Design review of the part built by this model. Coordinates are the model's own, in mm. Face numbers are marked on the shaded views. Round coordinates to 2 decimals unless told otherwise and drop trailing zeros. Loops run counter-clockwise (first coordinate to the right, second up) from the corner with the lowest first, then second, coordinate; pieces in that order, holes last. Notation, with made-up numbers: (80.25, -33) - (99.25, -33) arc R16 cw to (99.25, -21) - close; hole circle Ø8 at (60, 23.5). An arc over 180 degrees is marked (long way). Return JSON: item names as keys, results as strings. Group by question number.
(1) We need section A-A, the plane y = 15. Write out the cut boundary in (x, z), and give its area (3 significant figures).
(2) We need section C-C, the plane z = 45. Write out the cut boundary in (x, y), and give its area (3 significant figures).
(3) We need section D-D, the plane z = -32. Write out the cut boundary in (x, y), and give its area (3 significant figures).
(4) Wall thickness on L1, parallel to Z at x = 0.6, y = 30; L2, parallel to Y at x = 0.5, z = 45; L3, parallel to Z at x = 1.5, y = 17.5: over which ranges is each line inside the solid? List them lowest first. Write a range as [from, to].
(5) We need section B-B, the plane z = 20. Write out the cut boundary in (x, y), and give its area (3 significant figures).
(6) Clearance check with flat-ended pins moving along their axes: pin 1 (4 mm diameter, centred on x = 5, y = 60, fed in from +Z); pin 2 (16.5 mm diameter, centred on y = 18.5, z = -22, fed in from +X); pin 3 (4 mm diameter, centred on x = 1.5, z = 45.5, fed in from +Y); pin 4 (5 mm diameter, centred on x = 6, z = 28.5, fed in from +Y). State where each tip first meets the part, or that it passes through.
(7) The part is to be moulded in two halves that separate along X. For the marked faces 1, 2 and 3, say which applies: pulls with the +X half, pulls with the -X half, needs draft (parallel to the pull), parting line crosses it, or undercut.
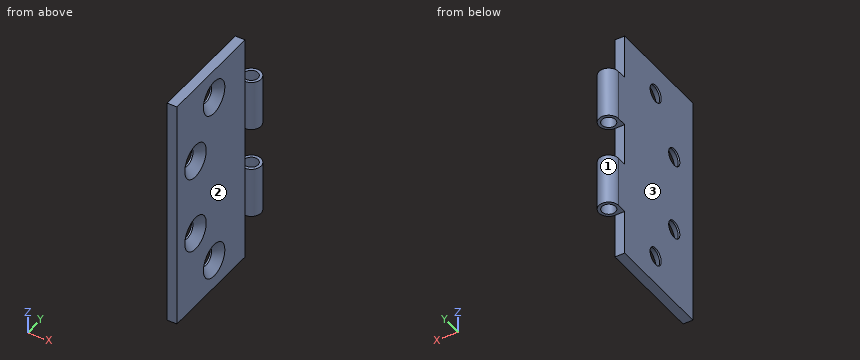
from build123d import *

# Parameters (mm, degrees)
SKETCH_1_W                 = 5
SKETCH_1_H                 = 60
EXTRUDE_1_DEPTH            = 60
SKETCH_2_R                 = 5
SKETCH_4_R                 = 3.5
CUT_EXTRUDE_1_DEPTH        = 137.839321834
HOLE_WIZARD_M81_AT_2_COUNT = 2
HOLE_WIZARD_M81_AT_2_PITCH = 29.154759474
CUT_EXTRUDE_2_DEPTH        = 89.600225733
CUT_EXTRUDE_2_DEPTH_BACK   = 89.600225733
SKETCH_7_W                 = 23
SKETCH_7_H                 = 10
SKETCH_7_W_2               = 22


with BuildPart() as part:
    # Эскиз1 → Вытянуть-Тонкостенный1 (new, symmetric)
    with BuildSketch(Plane.XY):
        with Locations((2.5, 30)):
            Rectangle(SKETCH_1_W, SKETCH_1_H)
    extrude(amount=EXTRUDE_1_DEPTH, both=True)

    # По траектории1: sweep along a curve in space
    with BuildLine() as sweep_1_path:
        Line((5, 60, 60), (5, 60, -60))
    # Эскиз2 → По траектории1 (sweep)
    with BuildSketch(Plane.XY.offset(60)):
        with Locations((5, 60)):
            Circle(SKETCH_2_R)
    sweep(path=sweep_1_path.line)

    # Эскиз4 → Вырез-Вытянуть1 (cut, through all)
    with BuildSketch(Plane.XY.offset(60)):
        with Locations((5, 60)):
            Circle(SKETCH_4_R)
    extrude(amount=-CUT_EXTRUDE_1_DEPTH, mode=Mode.SUBTRACT)

    # Эскиз5 → Зенковка для  винта с плоской головкой M81 (revolve, cut)
    with BuildSketch(Plane(origin=(5, 30, 45), x_dir=(0, 0, -1), z_dir=(0, 1, 0))):
        Polygon((0, 0), (0, 5), (4.5, 5), (4.5, 4.15), (8.65, 0), align=None)
    hole_wizard_m81 = revolve(axis=Axis((11.35, 30, 45), (-1, 0, 0)), mode=Mode.SUBTRACT)

    # Зенковка для  винта с плоской головкой M81 at 2: Зенковка для  винта с плоской головкой M81 ×2
    with Locations(*[Vector(0, -0.5144957554275265, -0.8574929257125442) * (i * HOLE_WIZARD_M81_AT_2_PITCH) for i in range(1, HOLE_WIZARD_M81_AT_2_COUNT)]):
        add(hole_wizard_m81, mode=Mode.SUBTRACT)

    # Зеркальное отражение1: Зенковка для  винта с плоской головкой M81 across plane
    add(hole_wizard_m81.mirror(Plane.XY), mode=Mode.SUBTRACT)

    # Зеркальное отражение1 copy 1 sketch → Зеркальное отражение1 copy 1 (revolve, cut)
    with BuildSketch(Plane(origin=(5, 15, -20), x_dir=(0, 0, 1), z_dir=(0, 1, 0))):
        Polygon((0, 0), (0, -5), (4.5, -5), (4.5, -4.15), (8.65, 0), align=None)
    revolve(axis=Axis((11.35, 15, -20), (1, 0, 0)), mode=Mode.SUBTRACT)

    # Эскиз7 → Вырез-Вытянуть2 (cut, two sides: drawn at the far end of the back side and taken through both)
    with BuildSketch(Plane(origin=(5, 0, 0), x_dir=(0, 0, -1), z_dir=(1, 0, 0)).offset(-CUT_EXTRUDE_2_DEPTH_BACK)):
        with Locations((48.5, 60)):
            Rectangle(SKETCH_7_W, SKETCH_7_H)
        with Locations((0, 60)):
            Rectangle(SKETCH_7_W_2, SKETCH_7_H)
        with Locations((-48.5, 60)):
            Rectangle(SKETCH_7_W, SKETCH_7_H)
    extrude(amount=CUT_EXTRUDE_2_DEPTH + CUT_EXTRUDE_2_DEPTH_BACK, mode=Mode.SUBTRACT)


solid = part.part
Solutions:
{
 "1": {"outline": "(0, -60) - (5, -60) - (5, -28.65) - (0.85, -24.5) - (0, -24.5) - close; (0, -15.5) - (0.85, -15.5) - (5, -11.35) - (5, 11.35) - (0.85, 15.5) - (0, 15.5) - close; (0, 24.5) - (0.85, 24.5) - (5, 28.65) - (5, 60) - (0, 60) - close", "area": "476 mm^2"},
 "2": {"outline": "(0, 0) - (5, 0) - (5, 21.35) - (0.85, 25.5) - (0, 25.5) - close; (0, 34.5) - (0.85, 34.5) - (5, 38.65) - (5, 55) - (0, 55) - close", "area": "213 mm^2"},
 "3": {"outline": "(0, 0) - (5, 0) - (5, 55) arc R5 ccw (long way) to (0, 60) - close; hole circle Ø7 at (5, 60)", "area": "320 mm^2"},
 "4": {"L1": "[-60, -49.5], [-40.5, 40.5], [49.5, 60]", "L2": "[0, 25.5], [34.5, 55]", "L3": "[-60, -24.5], [-15.5, 15.5], [24.5, 60]"},
 "5": {"outline": "(0, 0) - (5, 0) - (5, 6.35) - (0.85, 10.5) - (0, 10.5) - close; (0, 19.5) - (0.85, 19.5) - (5, 23.65) - (5, 55) arc R5 ccw (long way) to (0, 60) - close; hole circle Ø7 at (5, 60)", "area": "258 mm^2"},
 "6": {"pin 1": "through", "pin 2": "x = 5", "pin 3": "y = 55", "pin 4": "y = 65"},
 "7": {"face 1": "parting line crosses it", "face 2": "pulls with the +X half", "face 3": "pulls with the -X half"}
}
